from build123d import *

# Parameters (mm, degrees)
SKETCH1_W           = 6.25
SKETCH1_H           = 6
BOSS_EXTRUDE1_DEPTH = 0.71
BOSS_EXTRUDE2_DEPTH = 0.06
SKETCH3_W           = 1.25
SKETCH3_H           = 1.75
CUT_EXTRUDE1_DEPTH  = 1.71


with BuildPart() as part:
    # Sketch1 → Boss-Extrude1 (new body)
    with BuildSketch(Plane(origin=(0, 0, 0), x_dir=(1, 0, 0), z_dir=(0, 1, 0))):
        Rectangle(SKETCH1_W, SKETCH1_H)
    extrude(amount=BOSS_EXTRUDE1_DEPTH)

    # Sketch2 → Boss-Extrude2 (add)
    with BuildSketch(Plane(origin=(0, 0.71, 0), x_dir=(1, 0, 0), z_dir=(0, 1, 0))):
        Polygon((3.125, 3), (-3.125, 3), (-3.125, -3), (0.125, -3), (0.125, -1.5), (3.125, -1.5), (3.125, -1), (1.875, -1), (1.875, 0.75), (3.125, 0.75), align=None)
    extrude(amount=BOSS_EXTRUDE2_DEPTH)

    # Sketch3 → Cut-Extrude1 (cut, through all)
    with BuildSketch(Plane(origin=(0, 0.71, 0), x_dir=(1, 0, 0), z_dir=(0, 1, 0))):
        with Locations((2.5, -0.125)):
            Rectangle(SKETCH3_W, SKETCH3_H)
    extrude(amount=-CUT_EXTRUDE1_DEPTH, mode=Mode.SUBTRACT)


solid = part.part
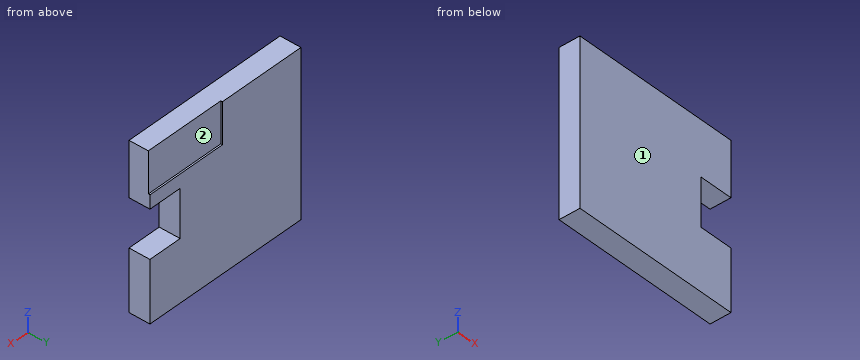
Verification items for the finished model (mm, model axes). Face numbers are marked on the shaded views. A direction names the side the tool comes from. Give positions to 0.01 mm unless a question says otherwise; leave off trailing zeros. Loops run counter-clockwise (first coordinate to the right, second up) from the corner with the lowest first, then second, coordinate; pieces in that order, holes last.
1. Cross-section at A-A on y = 0.35. Record the cut outline in (x, z) (3 decimals), and give its area (3 significant figures).
Derived:
outline: (-3.125, -3) - (3.125, -3) - (3.125, -0.75) - (1.875, -0.75) - (1.875, 1) - (3.125, 1) - (3.125, 3) - (-3.125, 3) - close
area: 35.3 mm2
2. Go/stop test with a flat-tipped pin: P1, Ø0.8, axis at x = 2, z = 2, coming from the +Y side. Record where the tip stops, or that it passes through.
Derived:
P1: stops at y = 0.71
3. Cross-section at B-B on z = 2.45. Record the cut outline in (x, y) (3 decimals).
Derived:
outline: (-3.125, 0) - (3.125, 0) - (3.125, 0.71) - (0.125, 0.71) - (0.125, 0.77) - (-3.125, 0.77) - close
4. Tool access check on the marked faces 1 and 2. Record the directions out of +Z, -Z, +X, -X, +Y, -Y that give a thin tool (end or side, any length) a straight path to the whole face; none if there is none.
Derived:
face 1: +Z, -Z, +X, -X, -Y
face 2: +Z, +X, +Y
5. Cross-section at C-C on x = 0.5. Record the cut outline in (y, z), and give its area (3 significant figures).
Derived:
outline: (0, -3) - (0.77, -3) - (0.77, 1.5) - (0.71, 1.5) - (0.71, 3) - (0, 3) - close
area: 4.53 mm2
6. Material ranges on probe 1 along Z at (x, y) = (2.75, 0.1); probe 2 along X at (y, z) = (0.7, -0.15) (3 decimals), recorded low to high.
Derived:
probe 1: z = -3 to -0.75, 1 to 3
probe 2: x = -3.125 to 1.875
